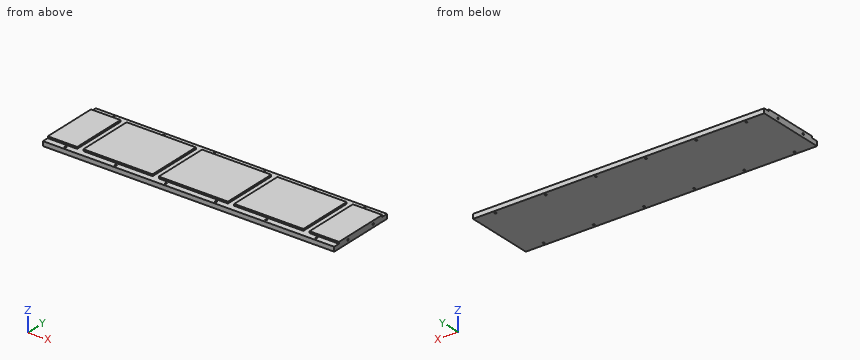
from build123d import *

# Parameters (mm, degrees)
SKETCH1_W                    = 842
SKETCH1_H                    = 200
BOSS_EXTRUDE1_DEPTH          = 18
SKETCH2_W                    = 5
SKETCH2_H                    = 18
CUT_EXTRUDE1_DEPTH           = 849.108483627
SKETCH3_W                    = 18
SKETCH3_H                    = 294.880521595
CUT_EXTRUDE2_DEPTH           = 5
F_5_0_5_DIAMETER_HOLE1_D     = 5
F_5_0_5_DIAMETER_HOLE2_D     = 5
F_5_0_5_DIAMETER_HOLE2_DEPTH = 45
F_5_0_5_DIAMETER_HOLE2_TIP   = 1.502151548
F_5_0_5_DIAMETER_HOLE3_D     = 5
F_5_0_5_DIAMETER_HOLE3_DEPTH = 45
F_5_0_5_DIAMETER_HOLE3_TIP   = 1.502151548


with BuildPart() as part:
    # Sketch1 → Boss-Extrude1 (new body)
    with BuildSketch(Plane.XY):
        Rectangle(SKETCH1_W, SKETCH1_H)
    extrude(amount=BOSS_EXTRUDE1_DEPTH)

    # Sketch2 → Cut-Extrude1 (cut, through all)
    with BuildSketch(Plane(origin=(421, 0, 0), x_dir=(0, 0, -1), z_dir=(1, 0, 0))):
        with Locations((-15.5, 91)):
            Rectangle(SKETCH2_W, SKETCH2_H)
        with Locations((-15.5, -91)):
            Rectangle(SKETCH2_W, SKETCH2_H)
    extrude(amount=-CUT_EXTRUDE1_DEPTH, mode=Mode.SUBTRACT)

    # Sketch3 → Cut-Extrude2 (cut)
    with BuildSketch(Plane.XY.offset(18)):
        with Locations((-327, -12.793720482)):
            Rectangle(SKETCH3_W, SKETCH3_H)
        with Locations((-109, -12.793720482)):
            Rectangle(SKETCH3_W, SKETCH3_H)
        with Locations((109, -12.793720482)):
            Rectangle(SKETCH3_W, SKETCH3_H)
        with Locations((327, -12.793720482)):
            Rectangle(SKETCH3_W, SKETCH3_H)
    extrude(amount=-CUT_EXTRUDE2_DEPTH, mode=Mode.SUBTRACT)

    # Ø5.0 (5) Diameter Hole1 (through all)
    with Locations(Plane.XY.offset(13)):
        with Locations((-362.5, 91), (-217.5, 91), (-72.5, 91), (72.5, 91), (217.5, 91), (362.5, 91), (-362.5, -91), (217.5, -91), (362.5, -91), (-217.5, -91), (-72.5, -91), (72.5, -91)):
            Hole(F_5_0_5_DIAMETER_HOLE1_D / 2)

    # Ø5.0 (5) Diameter Hole2
    with Locations(Plane(origin=(421, 0, 0), x_dir=(0, 0, -1), z_dir=(1, 0, 0))):
        with Locations((-9, 48), (-9, -48)):
            Hole(F_5_0_5_DIAMETER_HOLE2_D / 2, depth=F_5_0_5_DIAMETER_HOLE2_DEPTH)
            with Locations((0, 0, -(F_5_0_5_DIAMETER_HOLE2_DEPTH + F_5_0_5_DIAMETER_HOLE2_TIP / 2))):  # 118° drill point
                Cone(0, F_5_0_5_DIAMETER_HOLE2_D / 2, F_5_0_5_DIAMETER_HOLE2_TIP, mode=Mode.SUBTRACT)

    # Ø5.0 (5) Diameter Hole3
    with Locations(Plane.ZY.offset(421)):
        with Locations((9, 48), (9, -48)):
            Hole(F_5_0_5_DIAMETER_HOLE3_D / 2, depth=F_5_0_5_DIAMETER_HOLE3_DEPTH)
            with Locations((0, 0, -(F_5_0_5_DIAMETER_HOLE3_DEPTH + F_5_0_5_DIAMETER_HOLE3_TIP / 2))):  # 118° drill point
                Cone(0, F_5_0_5_DIAMETER_HOLE3_D / 2, F_5_0_5_DIAMETER_HOLE3_TIP, mode=Mode.SUBTRACT)


solid = part.part
The model under review builds one solid part; all positions refer to its coordinate system, in mm. Round coordinates to 2 decimals unless told otherwise and drop trailing zeros. Order: outer loops, then holes, each group sorted by start corner. A loop starts at its lowest first (then second) coordinate and runs counter-clockwise, first axis right, second up. Notation, with made-up numbers: (-5, -9) -> (50, -9) arc R25 cw to (50, 10) -> close; hole circle Ø5 at (18.25, 51). An arc over 180 degrees is marked (long way). Write item = value, one per line. Start each with the question number.
Item 1: Consider section A-A on x = -280. Write out the cut boundary in (y, z), plus the area to 3 significant figures.
Item 2: Consider section B-B on y = -2. Write out the cut boundary in (x, z), plus the area to 3 significant figures.
Item 3: Clearance check with flat-ended pins moving along their axes: pin 1 Ø8 at (x, y) = (-72.5, -91) entering from -Z; pin 2 Ø4 at (x, z) = (-378, 16) entering from -Y; pin 3 Ø1.5 at (x, z) = (-11.5, 15) entering from +Y. State where each tip first meets the part, or that it passes through.
Item 4: For line 1 along X through (y, z) = (-5, 15.5); line 2 along Y through (x, z) = (217.5, 9.5); line 3 along Y through (x, z) = (-408, 9), list the stretches that pass through material, from the lowest coordinate up.
Conclusion:
q1.outline = (-100, 0) -> (100, 0) -> (100, 13) -> (82, 13) -> (82, 18) -> (-82, 18) -> (-82, 13) -> (-100, 13) -> close
q1.area = 3,420 mm2
q2.outline = (-421, 0) -> (421, 0) -> (421, 18) -> (336, 18) -> (336, 13) -> (318, 13) -> (318, 18) -> (118, 18) -> (118, 13) -> (100, 13) -> (100, 18) -> (-100, 18) -> (-100, 13) -> (-118, 13) -> (-118, 18) -> (-318, 18) -> (-318, 13) -> (-336, 13) -> (-336, 18) -> (-421, 18) -> close
q2.area = 14,800 mm2
q3.pin_1 = 0
q3.pin_2 = -82
q3.pin_3 = 82
q4.line_1 = -421 to -336, -318 to -118, -100 to 100, 118 to 318, 336 to 421
q4.line_2 = -100 to -93.5, -88.5 to 88.5, 93.5 to 100
q4.line_3 = -100 to -50.5, -45.5 to 45.5, 50.5 to 100
